Can you work these out from the model? Positions are in its coordinate system, mm. A direction names the side the tool comes from. Round coordinates to 2 decimals unless told otherwise and drop trailing zeros. Order: outer loops, then holes, each group sorted by start corner. A loop starts at its lowest first (then second) coordinate and runs counter-clockwise, first axis right, second up. Notation, with made-up numbers: (46.25, 71.25) -> (77.25, 71.25) arc R26 cw to (77.25, 86.25) -> close; hole circle Ø1 at (-18, -14). An arc over 180 degrees is marked (long way). One line per item, written item: value.
```python
from build123d import *

# Parameters (mm, degrees)
F0_R     = 25
F1_DEPTH = 3


with BuildPart() as f1:
    # F0 (on Top) → F1 (new body)
    with BuildSketch(Plane.XY):
        with BuildLine():
            Line((30, 1.5), (34.967842, 1.5))
            ThreePointArc((34.967842, 1.5), (34.327485, 6.828161), (32.880099, 11.995795))
            Line((32.880099, 11.995795), (28.290411, 10.094684))
            Line((28.290411, 10.094684), (27.142361, 12.866322))
            Line((27.142361, 12.866322), (31.732049, 14.767433))
            ThreePointArc((31.732049, 14.767433), (29.101436, 19.444958), (25.786659, 23.665338))
            Line((25.786659, 23.665338), (22.273864, 20.152543))
            Line((22.273864, 20.152543), (20.152543, 22.273864))
            Line((20.152543, 22.273864), (23.665338, 25.786659))
            ThreePointArc((23.665338, 25.786659), (19.444958, 29.101436), (14.767433, 31.732049))
            Line((14.767433, 31.732049), (12.866322, 27.142361))
            Line((12.866322, 27.142361), (10.094684, 28.290411))
            Line((10.094684, 28.290411), (11.995795, 32.880099))
            ThreePointArc((11.995795, 32.880099), (6.828161, 34.327485), (1.5, 34.967842))
            Line((1.5, 34.967842), (1.5, 30))
            Line((1.5, 30), (-1.5, 30))
            Line((-1.5, 30), (-1.5, 34.967842))
            ThreePointArc((-1.5, 34.967842), (-6.828161, 34.327485), (-11.995795, 32.880099))
            Line((-11.995795, 32.880099), (-10.094684, 28.290411))
            Line((-10.094684, 28.290411), (-12.866322, 27.142361))
            Line((-12.866322, 27.142361), (-14.767433, 31.732049))
            ThreePointArc((-14.767433, 31.732049), (-19.444958, 29.101436), (-23.665338, 25.786659))
            Line((-23.665338, 25.786659), (-20.152543, 22.273864))
            Line((-20.152543, 22.273864), (-22.273864, 20.152543))
            Line((-22.273864, 20.152543), (-25.786659, 23.665338))
            ThreePointArc((-25.786659, 23.665338), (-29.101436, 19.444958), (-31.732049, 14.767433))
            Line((-31.732049, 14.767433), (-27.142361, 12.866322))
            Line((-27.142361, 12.866322), (-28.290411, 10.094684))
            Line((-28.290411, 10.094684), (-32.880099, 11.995795))
            ThreePointArc((-32.880099, 11.995795), (-34.327485, 6.828161), (-34.967842, 1.5))
            Line((-34.967842, 1.5), (-30, 1.5))
            Line((-30, 1.5), (-30, -1.5))
            Line((-30, -1.5), (-34.967842, -1.5))
            ThreePointArc((-34.967842, -1.5), (-34.327485, -6.828161), (-32.880099, -11.995795))
            Line((-32.880099, -11.995795), (-28.290411, -10.094684))
            Line((-28.290411, -10.094684), (-27.142361, -12.866322))
            Line((-27.142361, -12.866322), (-31.732049, -14.767433))
            ThreePointArc((-31.732049, -14.767433), (-29.101436, -19.444958), (-25.786659, -23.665338))
            Line((-25.786659, -23.665338), (-22.273864, -20.152543))
            Line((-22.273864, -20.152543), (-20.152543, -22.273864))
            Line((-20.152543, -22.273864), (-23.665338, -25.786659))
            ThreePointArc((-23.665338, -25.786659), (-19.444958, -29.101436), (-14.767433, -31.732049))
            Line((-14.767433, -31.732049), (-12.866322, -27.142361))
            Line((-12.866322, -27.142361), (-10.094684, -28.290411))
            Line((-10.094684, -28.290411), (-11.995795, -32.880099))
            ThreePointArc((-11.995795, -32.880099), (-6.828161, -34.327485), (-1.5, -34.967842))
            Line((-1.5, -34.967842), (-1.5, -30))
            Line((-1.5, -30), (0, -30))
            Line((0, -30), (1.5, -30))
            Line((1.5, -30), (1.5, -34.967842))
            ThreePointArc((1.5, -34.967842), (6.828161, -34.327485), (11.995795, -32.880099))
            Line((11.995795, -32.880099), (10.094684, -28.290411))
            Line((10.094684, -28.290411), (12.866322, -27.142361))
            Line((12.866322, -27.142361), (14.767433, -31.732049))
            ThreePointArc((14.767433, -31.732049), (19.444958, -29.101436), (23.665338, -25.786659))
            Line((23.665338, -25.786659), (20.152543, -22.273864))
            Line((20.152543, -22.273864), (22.273864, -20.152543))
            Line((22.273864, -20.152543), (25.786659, -23.665338))
            ThreePointArc((25.786659, -23.665338), (29.101436, -19.444958), (31.732049, -14.767433))
            Line((31.732049, -14.767433), (27.142361, -12.866322))
            Line((27.142361, -12.866322), (28.290411, -10.094684))
            Line((28.290411, -10.094684), (32.880099, -11.995795))
            ThreePointArc((32.880099, -11.995795), (34.327485, -6.828161), (34.967842, -1.5))
            Line((34.967842, -1.5), (30, -1.5))
            Line((30, -1.5), (30, 1.5))
        make_face()
        Circle(F0_R, mode=Mode.SUBTRACT)
    extrude(amount=F1_DEPTH)


solid = f1.part
```
Q1. On a 3-axis mill with a long thin cutter (end or side, diameter ignored), from which of +Z, -Z, +X, -X, +Y, -Y can I reach the whole of each face in a straight line? I mean faces 5 (the face through (13.8, -29.4, 1.5)), 6 (the face through (30.55, -11.03, 1.48)), 7 (the face through (-29.47, 13.83, 1.48)). Say none if no direction works.
Answers below:
face 5: +Z, -Z, -Y
face 6: +Z, -Z
face 7: +Z, -Z, -X
Q2. We'd pull the mould along Y, two halves only. Please class faces 1 (the face through (-30.55, 11.03, 1.48)), 2 (the face through (1.5, 33, 1)), 3 (the face through (6.902, 34.313, 1.479)), 4 (the face through (-6.902, -34.313, 1.479)): released by +Y, released by -Y, zero draft, split by the parting line, or undercut.
Answers below:
face 1: undercut
face 2: zero draft
face 3: released by +Y
face 4: released by -Y
Q3. Please list where these lines run through material, in increasing order: line 1 along Y through (x, z) = (0, 2.4); line 2 along Y through (x, z) = (-11.5, 2.1); line 3 along Y through (x, z) = (-21.5, 0.6).
Answers below:
line 1: -30 to -25, 25 to 30
line 2: -33.06 to -31.68, -27.71 to -22.2, 22.2 to 27.71, 31.68 to 33.06
line 3: -27.62 to -23.62, -20.93 to -12.76, 12.76 to 20.93, 23.62 to 27.62
Q4. I want a section at A-A on x = 0. List the corners of the cut face in (y, z) for me, plus the area to 3 significant figures.
Answers below:
outline: (-30, 0) -> (-25, 0) -> (-25, 3) -> (-30, 3) -> close; (25, 0) -> (30, 0) -> (30, 3) -> (25, 3) -> close
area: 30.0 mm^2
Q5. Will these pins go through, and if not, where does the flat tip stop? pin 1 Ø1.5 at (x, z) = (-33.5, 2) entering from +Y; pin 2 Ø0.9 at (y, z) = (31.5, 1) entering from -X; pin 3 Ø0.9 at (y, z) = (-32, 1) entering from +X; pin 4 Ø4 at (x, y) = (-14.5, 16.5) entering from +Z.
Answers below:
pin 1: y = 12
pin 2: x = -16.15
pin 3: x = 15.15
pin 4: through
